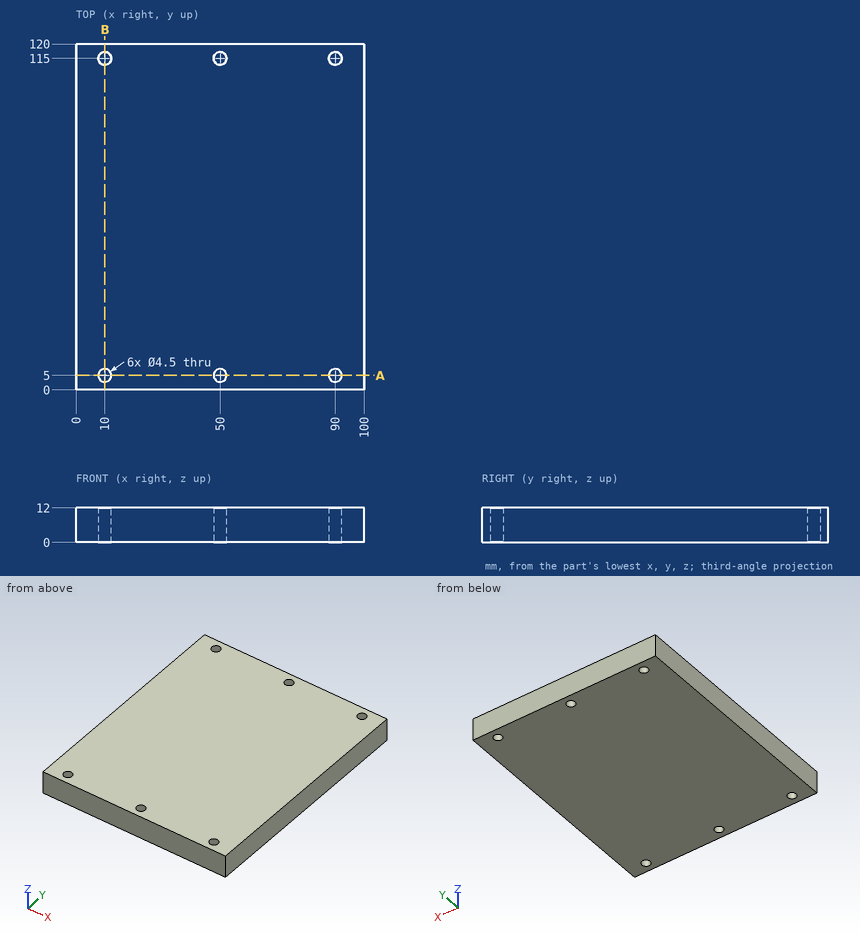
For this review, use the dimensioned drawing (mm, ordinates from the lowest corner) and the shaded views. Round coordinates to 2 decimals unless told otherwise and drop trailing zeros. Loops run counter-clockwise (first coordinate to the right, second up) from the corner with the lowest first, then second, coordinate; pieces in that order, holes last. Notation, with made-up numbers: M 71,13 L 81,13 A25 cw 81,40 Z; hole C -40,-23 d9. An arc over 180 degrees is marked long. Answer as CSV lines item,"result".
1. To check wall thickness, follow L1, parallel to Y at x = 90, z = 5.5; L2, parallel to X at y = 115, z = 4.5; L3, parallel to Y at x = 49, z = 9. State the ranges of each line that lie inside material, in increasing order. Write a range as [from, to].
Outcome:
L1,"y = [0, 2.75], [7.25, 112.75], [117.25, 120]"
L2,"x = [0, 7.75], [12.25, 47.75], [52.25, 87.75], [92.25, 100]"
L3,"y = [0, 2.98], [7.02, 112.98], [117.02, 120]"
2. Insertion check: pin 1 Ø2.5 at (x, y) = (50, 115) entering from -Z. The pin has a flat end and moves straight along its axis. Give the tip position at first contact, or say it passes through.
Outcome:
pin 1,"passes through"
3. We need section B-B (x = 10). Give the boundary of the cut face in (y, z).
Outcome:
outline,"M 0,0 L 2.75,0 L 2.75,12 L 0,12 Z; M 7.25,0 L 112.75,0 L 112.75,12 L 7.25,12 Z; M 117.25,0 L 120,0 L 120,12 L 117.25,12 Z"
4. We need section A-A (y = 5). Give the boundary of the cut face in (x, z), plus the area to 3 significant figures.
Outcome:
outline,"M 0,0 L 7.75,0 L 7.75,12 L 0,12 Z; M 12.25,0 L 47.75,0 L 47.75,12 L 12.25,12 Z; M 52.25,0 L 87.75,0 L 87.75,12 L 52.25,12 Z; M 92.25,0 L 100,0 L 100,12 L 92.25,12 Z"
area,"1,040 mm2"
